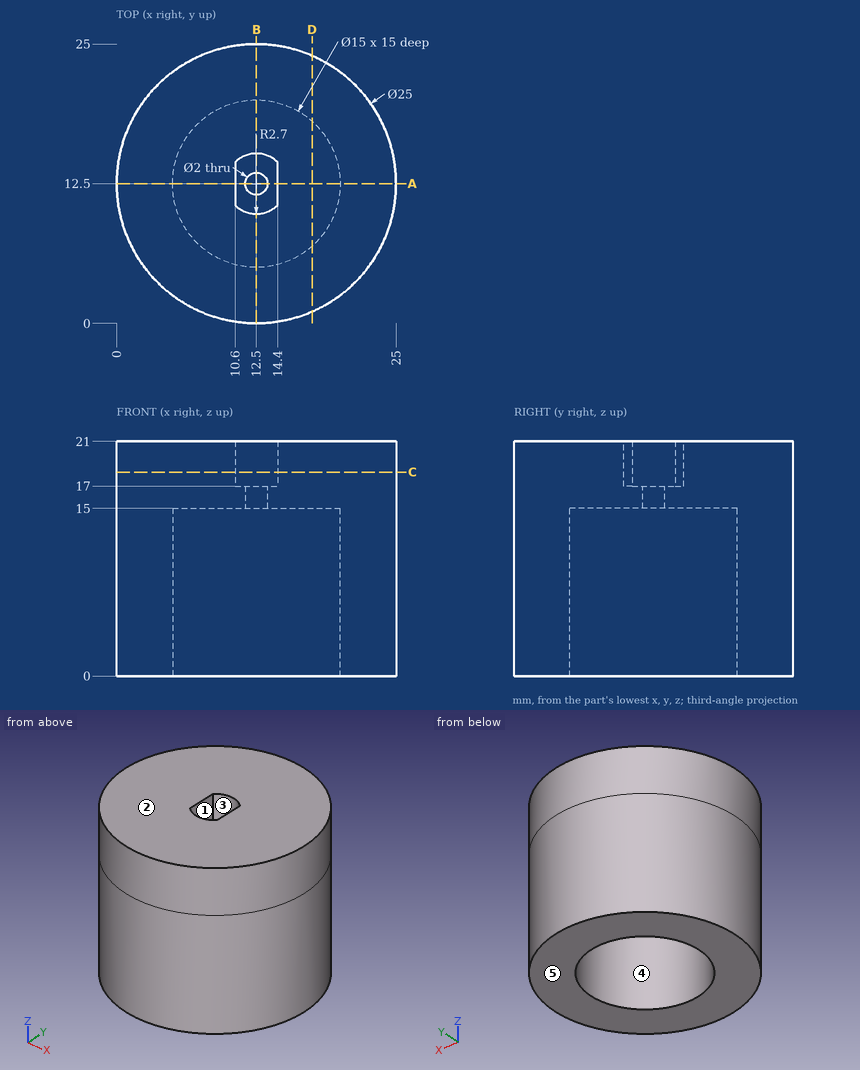
Here's the drawing with two shaded views (mm, measured from the low corner). I have some questions. A direction names the side the tool comes from. Give positions to 0.01 mm unless a question says otherwise; leave off trailing zeros. Order: outer loops, then holes, each group sorted by start corner. A loop starts at its lowest first (then second) coordinate and runs counter-clockwise, first axis right, second up. Notation, with made-up numbers: (-26.75, 29.5) -> (24.25, 29.5) arc R15 ccw to (24.25, 51.5) -> close; hole circle Ø7 at (19.25, 44). An arc over 180 degrees is marked (long way). Use a Markdown table: item, result. Add a question column.
Item 1: For the marked faces 1 and 2, which set-ups out of +Z, -Z, +X, -X, +Y, -Y let a thin tool reach every point of the face, with its end or its side?
Item 2: Imagine slicing it at B-B on x = 12.5. Please give me the cut outline in (y, z).
Item 3: Imagine slicing it at A-A on y = 12.5. Please give me the cut outline in (x, z).
Item 4: I need wall thicknesses on line 1 (Y direction, x = 12.5, z = 3.5); line 2 (X direction, y = 22.5, z = 15); line 3 (Z direction, x = 16.75, y = 9.75). Which ranges of each line are inside material? Lowest first, please.
Item 5: If we mould it in two halves opening along Y, with no side actions, what happens to the marked faces 3, 4 and 5? For each: pulls with the +Y half, pulls with the -Y half, needs draft (parallel to the pull), parting line crosses it, or undercut.
Item 6: Imagine slicing it at D-D on x = 17.5. Please give me the cut outline in (y, z).
Item 7: Imagine slicing it at C-C on z = 18.25. Please give me the cut outline in (x, y).
Item 8: Will these pins go through, and if not, where does the flat tip stop? pin 1 (2 mm diameter, centred on y = 16.5, z = 15, fed in from +X); pin 2 (1.5 mm diameter, centred on x = 8.5, z = 5, fed in from -Y); pin 3 (1.5 mm diameter, centred on y = 18, z = 15.5, fed in from +X); pin 4 (1.2 mm diameter, centred on x = 12.5, y = 12.5, fed in from -Z).
Data:
| question | item | result |
|---|---|---|
| 1 | face 1 | +Z |
| 1 | face 2 | +Z, +X, -X, +Y, -Y |
| 2 | outline | (0, 0) -> (5, 0) -> (5, 15) -> (11.5, 15) -> (11.5, 17) -> (9.8, 17) -> (9.8, 21) -> (0, 21) -> close; (13.5, 15) -> (20, 15) -> (20, 0) -> (25, 0) -> (25, 21) -> (15.2, 21) -> (15.2, 17) -> (13.5, 17) -> close |
| 3 | outline | (0, 0) -> (5, 0) -> (5, 15) -> (11.5, 15) -> (11.5, 17) -> (10.6, 17) -> (10.6, 21) -> (0, 21) -> close; (13.5, 15) -> (20, 15) -> (20, 0) -> (25, 0) -> (25, 21) -> (14.4, 21) -> (14.4, 17) -> (13.5, 17) -> close |
| 4 | line 1 | y = 0 to 5, 20 to 25 |
| 4 | line 2 | x = 5 to 20 |
| 4 | line 3 | z = 15 to 21 |
| 5 | face 3 | undercut |
| 5 | face 4 | undercut |
| 5 | face 5 | needs draft |
| 6 | outline | (1.04, 0) -> (6.91, 0) -> (6.91, 15) -> (18.09, 15) -> (18.09, 0) -> (23.96, 0) -> (23.96, 21) -> (1.04, 21) -> close |
| 7 | outline | circle Ø25 at (12.5, 12.5); hole (10.6, 10.58) arc R2.7 ccw to (14.4, 10.58) -> (14.4, 14.42) arc R2.7 ccw to (10.6, 14.42) -> close |
| 8 | pin 1 | stops at x = 24.63 |
| 8 | pin 2 | stops at y = 0.43 |
| 8 | pin 3 | stops at x = 24.06 |
| 8 | pin 4 | passes through |
